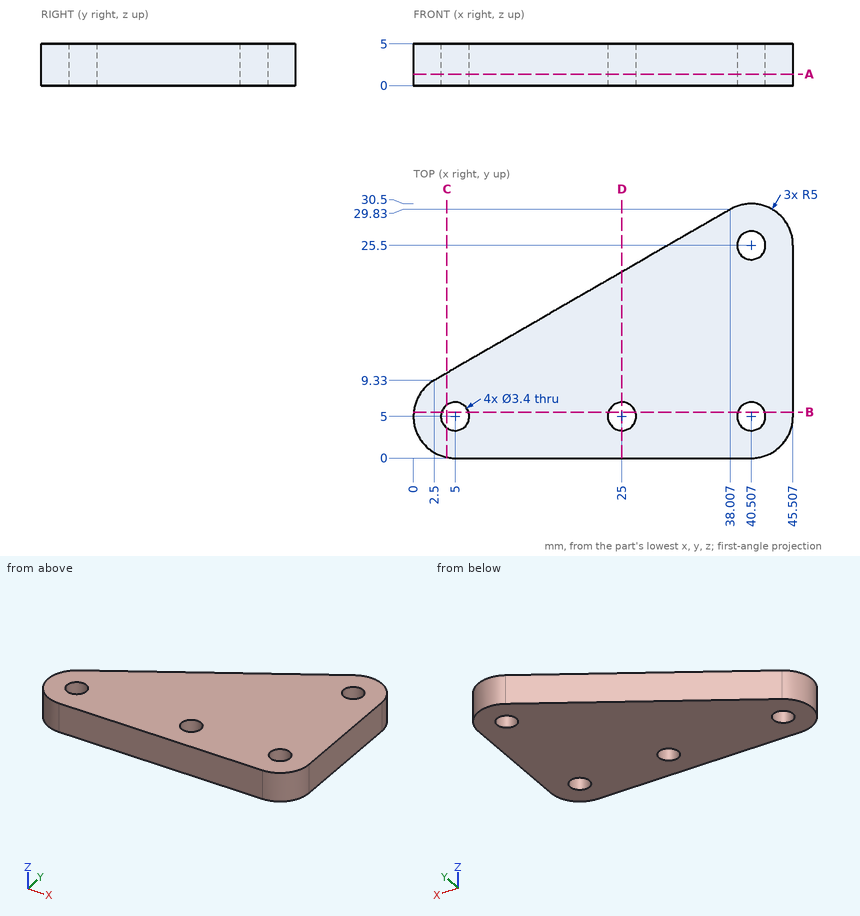
Geometry: see drawing. Coordinates: mm, zero at the bounding-box minimum. Coordinates: 2 decimals unless noted, no trailing zeros. Order: outer loops, then holes, each group sorted by start corner. A loop starts at its lowest first (then second) coordinate and runs counter-clockwise, first axis right, second up. Notation, with made-up numbers: (75, -17) -> (121, -17) arc R27 ccw to (121, 22) -> close; hole circle Ø5 at (-4.5, 27.25). An arc over 180 degrees is marked (long way). Write each question's results on one line, items separated by ' | '. Start each with the question number.
1) Cut plane D-D, the plane x = 25. Output: boundary loops of the cut face in (y, z).
2) Cut plane B-B, the plane y = 5.5. Output: boundary loops of the cut face in (x, z) (3 decimals), and give its area (3 significant figures).
3) Material intervals for line 1 along X through (y, z) = (26.5, 3.15) (1 decimal); line 2 along Y through (x, z) = (5, 3.3); line 3 along X through (y, z) = (27, 1.85) (1 decimal), sorted ascending.
4) First-contact query: pin 1 (1.5 mm diameter, centred on y = 27, z = 4, fed in from +X); pin 2 (1 mm diameter, centred on x = 31.5, z = 1, fed in from +Y); pin 3 (2.5 mm diameter, centred on x = 5, y = 5, fed in from +Z); pin 4 (1 mm diameter, centred on y = 17.5, z = 2, fed in from -X) (1 decimal). Flat tips, straight axial feed; report the tip coordinate or a pass-through.
5) Cut plane A-A, the plane z = 1.4. Output: boundary loops of the cut face in (x, y), and give its area (3 significant figures).
6) Cut plane C-C, the plane x = 4. Output: boundary loops of the cut face in (y, z) (3 decimals).
Checks:
1) outline: (0, 0) -> (3.3, 0) -> (3.3, 5) -> (0, 5) -> close; (6.7, 0) -> (22.32, 0) -> (22.32, 5) -> (6.7, 5) -> close
2) outline: (0.025, 0) -> (3.375, 0) -> (3.375, 5) -> (0.025, 5) -> close; (6.625, 0) -> (23.375, 0) -> (23.375, 5) -> (6.625, 5) -> close; (26.625, 0) -> (38.882, 0) -> (38.882, 5) -> (26.625, 5) -> close; (42.132, 0) -> (45.507, 0) -> (45.507, 5) -> (42.132, 5) -> close | area: 179 mm^2
3) line 1: 32.2 to 39.1, 41.9 to 45.4 | line 2: 0 to 3.3, 6.7 to 10.77 | line 3: 33.1 to 39.7, 41.3 to 45.3
4) pin 1: x = 45.45 | pin 2: y = 26.36 | pin 3: through | pin 4: x = 15.8
5) outline: (2.5, 9.33) arc R5 ccw to (5, 0) -> (40.51, 0) arc R5 ccw to (45.51, 5) -> (45.51, 25.5) arc R5 ccw to (38.01, 29.83) -> close; hole circle Ø3.4 at (5, 5); hole circle Ø3.4 at (25, 5); hole circle Ø3.4 at (40.51, 5); hole circle Ø3.4 at (40.51, 25.5) | area: 891 mm^2
6) outline: (0.101, 0) -> (3.625, 0) -> (3.625, 5) -> (0.101, 5) -> close; (6.375, 0) -> (10.196, 0) -> (10.196, 5) -> (6.375, 5) -> close
